```python
from build123d import *

# Parameters (mm, degrees)
SKETCH1_W           = 35
SKETCH1_H           = 30
SKETCH1_R           = 11
BOSS_EXTRUDE1_DEPTH = 6
SKETCH2_W           = 6
SKETCH2_H           = 17
BOSS_EXTRUDE2_DEPTH = 2
SKETCH3_W           = 6
SKETCH3_H           = 2.5
BOSS_EXTRUDE3_DEPTH = 11
CHAMFER1_SIZE       = 5
CHAMFER2_SIZE       = 2.5
CHAMFER3_SIZE       = 0.5


with BuildPart() as part:
    # Sketch1 → Boss-Extrude1 (new body)
    with BuildSketch(Plane.XY):
        Rectangle(SKETCH1_W, SKETCH1_H)
        Circle(SKETCH1_R, mode=Mode.SUBTRACT)
    extrude(amount=BOSS_EXTRUDE1_DEPTH)

    # Sketch2 → Boss-Extrude2 (add)
    with BuildSketch(Plane(origin=(0, 0, 0), x_dir=(-1, 0, 0), z_dir=(0, 0, -1))):
        with Locations((14.5, 6.5)):
            Rectangle(SKETCH2_W, SKETCH2_H)
        with Locations((-14.5, 6.5)):
            Rectangle(SKETCH2_W, SKETCH2_H)
    extrude(amount=BOSS_EXTRUDE2_DEPTH)

    # Sketch3 → Boss-Extrude3 (add)
    with BuildSketch(Plane(origin=(0, 0, -2), x_dir=(-1, 0, 0), z_dir=(0, 0, -1))):
        with Locations((14.5, -0.75)):
            Rectangle(SKETCH3_W, SKETCH3_H)
        with Locations((-14.5, -0.75)):
            Rectangle(SKETCH3_W, SKETCH3_H)
    extrude(amount=BOSS_EXTRUDE3_DEPTH)

    # Chamfer1
    chamfer1_edges = [part.edges().sort_by_distance(p)[0] for p in [
        (17.5, -15, 3),
        (-17.5, -15, 3),
        (-17.5, 15, 2),
        (17.5, 15, 2),
    ]]
    chamfer(chamfer1_edges, length=CHAMFER1_SIZE)

    # Chamfer2
    chamfer2_edges = [part.edges().sort_by_distance(p)[0] for p in [
        (-14.5, 0.5, -2),
        (14.5, 0.5, -2),
    ]]
    chamfer(chamfer2_edges, length=CHAMFER2_SIZE)

    # Chamfer3
    chamfer3_edges = [part.edges().sort_by_distance(p)[0] for p in [
        (-11.5, 6.5, 0),
        (11.5, 6.5, 0),
    ]]
    chamfer(chamfer3_edges, length=CHAMFER3_SIZE - 0.0001)  # a hair under: the kernel refuses the full size


solid = part.part
```
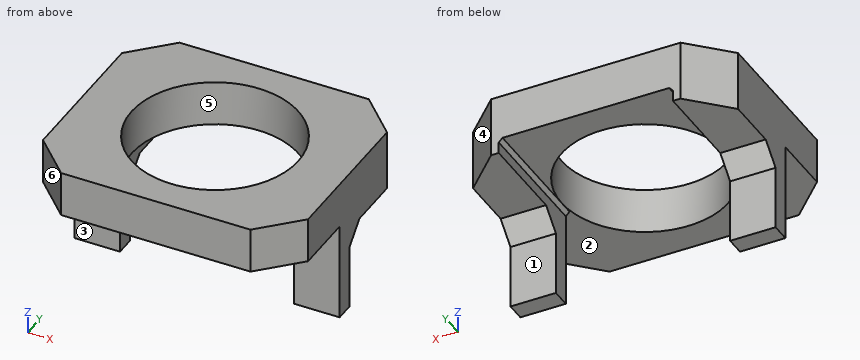
The model under review builds one solid part; all positions refer to its coordinate system, in mm. Face numbers are marked on the shaded views. A direction names the side the tool comes from. Round coordinates to 2 decimals unless told otherwise and drop trailing zeros. Order: outer loops, then holes, each group sorted by start corner. A loop starts at its lowest first (then second) coordinate and runs counter-clockwise, first axis right, second up. Notation, with made-up numbers: (53, -7.75) -> (64, -7.75) arc R26 cw to (64, 8.25) -> close; hole circle Ø10 at (19, 60). An arc over 180 degrees is marked (long way). One line per item, written item: value. Start each with the question number.
Q1. Mouldability with a two-part tool opening along Y and no side actions: class the marked faces 4, 5 and 6 as released by +Y, released by -Y, zero draft, split by the parting line, or undercut.
Q2. Wall thickness on line 1 (Y direction, x = 0, z = 2.6); line 2 (X direction, y = -0.5, z = -12); line 3 (Z direction, x = -14.5, y = -7): over which ranges is each line inside the solid? List them lowest first.
Q3. Take a section at D-D (x = 0). Write out the cut boundary in (y, z).
Q4. Take a section at A-A (z = -5.75). Write out the cut boundary in (x, y).
Q5. Machinability: for the marked faces 1, 2 and 3, which of the approach directions +Z, -Z, +X, -X, +Y, -Y give a long, thin tool a straight path to every point of the face, cutting with its end or side? Answer none if there is none.
Q6. Clearance check with flat-ended pins moving along their axes: pin 1 Ø3 at (x, z) = (16, -8) entering from +Y; pin 2 Ø5 at (y, z) = (-6, -10.5) entering from -X; pin 3 Ø5 at (x, z) = (12.5, -3) entering from -Y; pin 4 Ø6.5 at (x, y) = (14.5, 8) entering from -Z. State where each tip first meets the part, or that it passes through.
Q7. Take a section at C-C (z = 1.75). Write out the cut boundary in (x, y), and give its area (3 significant figures).
Reported:
1. face 4: released by +Y
1. face 5: undercut
1. face 6: released by -Y
2. line 1: y = -15 to -11, 11 to 15
2. line 2: x = -17.5 to -11.5, 11.5 to 17.5
2. line 3: z = 0 to 6
3. outline: (-15, 0) -> (-11, 0) -> (-11, 6) -> (-15, 6) -> close; (11, 0) -> (15, 0) -> (15, 6) -> (11, 6) -> close
4. outline: (-17.5, -2) -> (-11.5, -2) -> (-11.5, 0.5) -> (-17.5, 0.5) -> close; (11.5, -2) -> (17.5, -2) -> (17.5, 0.5) -> (11.5, 0.5) -> close
5. face 1: -Z, +X, -X, +Y
5. face 2: -Z, -Y
5. face 3: -Z, +X, -X, -Y
6. pin 1: stops at y = 0.5
6. pin 2: passes through
6. pin 3: stops at y = -2
6. pin 4: stops at z = -2
7. outline: (-17.5, -10) -> (-12.5, -15) -> (12.5, -15) -> (17.5, -10) -> (17.5, 10) -> (12.5, 15) -> (-12.5, 15) -> (-17.5, 10) -> close; hole circle Ø22 at (0, 0)
7. area: 620 mm2
